```python
from build123d import *

# Parameters (mm, degrees)
SKETCH_4_R          = 1.5
CUT_EXTRUDE_1_DEPTH = 10
CHAMFER_1_SIZE      = 0.5
CUT_EXTRUDE_2_DEPTH = 1


with BuildPart() as part:
    # 草图3 → 旋转1 (revolve)
    with BuildSketch(Plane(origin=(0, 0, 0), x_dir=(0, 0, -1), z_dir=(1, 0, 0)), mode=Mode.PRIVATE) as revolve_1_sk:
        Polygon((-7.5, 0), (0, 0), (0, -4), (-4.636363636, -4), (-16, -44), (-20, -44), align=None)
    revolve(revolve_1_sk.sketch.rotate(Axis((0, 28.450677981, 0), (0, 1, 0)), 180), axis=Axis((0, 28.450677981, 0), (0, 1, 0)))

    # 草图4 → 切除-拉伸1 (cut)
    with BuildSketch(Plane(origin=(0, 0, 0), x_dir=(1, 0, 0), z_dir=(0, 1, 0))):
        with Locations(Location((0, 0, 0), (0, 0, 270))):
            Circle(SKETCH_4_R)
    extrude(amount=-CUT_EXTRUDE_1_DEPTH, mode=Mode.SUBTRACT)

    # 倒角1
    chamfer_1_edges = [part.edges().sort_by_distance(p)[0] for p in [
        (0, -4, -1.5),
    ]]
    chamfer(chamfer_1_edges, length=CHAMFER_1_SIZE)

    # 草图5 → 切除-拉伸2 (cut)
    with BuildSketch(Plane(origin=(0, 0, 0), x_dir=(1, 0, 0), z_dir=(0, 1, 0))):
        Polygon((3.5, 0), (1.75, 3.031088913), (-1.75, 3.031088913), (-3.5, 0), (-1.75, -3.031088913), (1.75, -3.031088913), align=None)
    extrude(amount=-CUT_EXTRUDE_2_DEPTH, mode=Mode.SUBTRACT)


solid = part.part
```
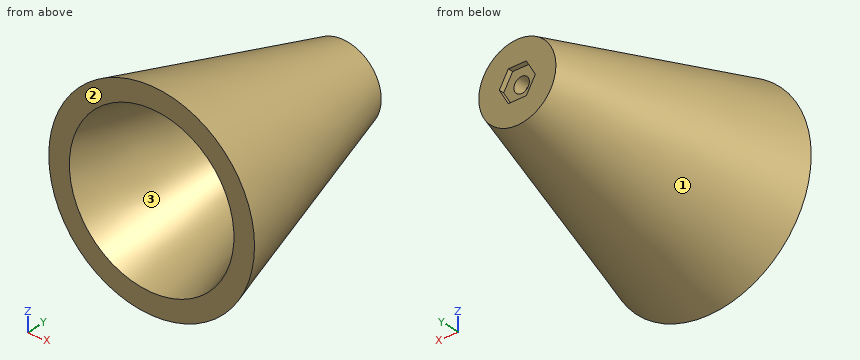
CAD build for the part. Positions are in the model's coordinates, mm. Face numbers are marked on the shaded views. Give positions to 0.01 mm unless a question says otherwise; leave off trailing zeros. Loops run counter-clockwise (first coordinate to the right, second up) from the corner with the lowest first, then second, coordinate; pieces in that order, holes last. Notation, with made-up numbers: (88, -24.75) - (132, -24.75) arc R6 cw to (132, -18.75) - close; hole circle Ø8 at (59.25, -27). An arc over 180 degrees is marked (long way). Put each result on its own line as item: value.
Q1. Slice it at B-B (y = -15.5). Give the cut face in (x, z), plus the area to 3 significant figures.
Filled in:
outline: circle Ø23.81 at (0, 0); hole circle Ø15.81 at (0, 0)
area: 249 mm²
Q2. Mould opens along X. For the marked faces 1, 2 and 3 say: pulls with the +X half, pulls with the -X half, needs draft (parallel to the pull), parting line crosses it, or undercut.
Filled in:
face 1: parting line crosses it
face 2: needs draft
face 3: undercut
Q3. Probe line 1 along X through (y, z) = (-10.5, 1); line 2 along Z through (x, y) = (5, -41); line 3 along X through (y, z) = (-40, 7). List the from-to ranges inside material, lowest first.
Filled in:
line 1: x = -10.44 to -6.41, 6.41 to 10.44
line 2: z = -18.48 to -14.3, 14.3 to 18.48
line 3: x = -17.52 to -13.11, 13.11 to 17.52
Q4. Slice it at C-C (y = -29). Give the cut face in (x, z).
Filled in:
outline: circle Ø31.48 at (0, 0); hole circle Ø23.48 at (0, 0)
Q5. Slice it at A-A (x = 0). Give the cut face in (y, z).
Filled in:
outline: (-44, -20) - (0, -7.5) - (0, -3.03) - (-1, -3.03) - (-1, -1.5) - (-3.5, -1.5) - (-4, -2) - (-4, -4.64) - (-44, -16) - close; (-44, 16) - (-4, 4.64) - (-4, 2) - (-3.5, 1.5) - (-1, 1.5) - (-1, 3.03) - (0, 3.03) - (0, 7.5) - (-44, 20) - close
Q6. Flat gauge pins, fed straight in: pin 1 (1.1 mm diameter, centred on x = 0, y = -0.5, fed in from +Z); pin 2 (2 mm diameter, centred on x = -1.5, z = -5.5, fed in from +Y); pin 3 (12 mm diameter, centred on y = -13, z = 10, fed in from +X); pin 4 (5 mm diameter, centred on y = -29, z = -3, fed in from -X). Where does each tip first touch, or does it go through?
Filled in:
pin 1: stops at z = 7.8
pin 2: stops at y = 0
pin 3: stops at x = 11.06
pin 4: stops at x = -16.27
